Check sheet for the drawn part. Datum: minimum x, y, z corner. Units: mm. A direction names the side the tool comes from. Give positions to 0.01 mm unless a question says otherwise; leave off trailing zeros. Order: outer loops, then holes, each group sorted by start corner. A loop starts at its lowest first (then second) coordinate and runs counter-clockwise, first axis right, second up. Notation, with made-up numbers: M 0,80.5 L 31,80.5 A32 cw 31,117.5 Z; hole C -17.75,-17 d7. An arc over 180 degrees is marked long. Put each result on its own line as item: value. Start each with the question number.
Q1. Section check C-C on z = 8. Record the cut outline in (x, y), then the cut area to 3 significant figures.
Q2. Section check B-B on x = 14. Record the cut outline in (y, z), then the cut area to 3 significant figures.
Q3. Access from +Z, -Z, +X, -X, +Y, -Y to the whole of each face (thin tool, end or side, straight path). Record for the marked faces 5 and 6.
Q4. Mould release check, pull along Z, two halves, no side actions. Record for the marked faces 1, 2, 3 and 4: +Z half, -Z half, draft (parallel to the pull), parting line (faces both ways), or undercut.
Q5. Material ranges on L1, parallel to X at y = 9, z = 23.25; L2, parallel to Y at x = 14, z = 27.05; L3, parallel to X at y = 2.5, z = 14.75, recorded low to high.
Q6. Section check A-A on z = 19.25. Record the cut outline in (x, y).
Q7. Section check D-D on x = 9.75. Record the cut outline in (y, z).
Q8. Go/stop test with a flat-tipped pin: pin 1 (6 mm diameter, centred on x = 12.5, z = 22, fed in from -Y). Record where the tip stops, or that it passes through.
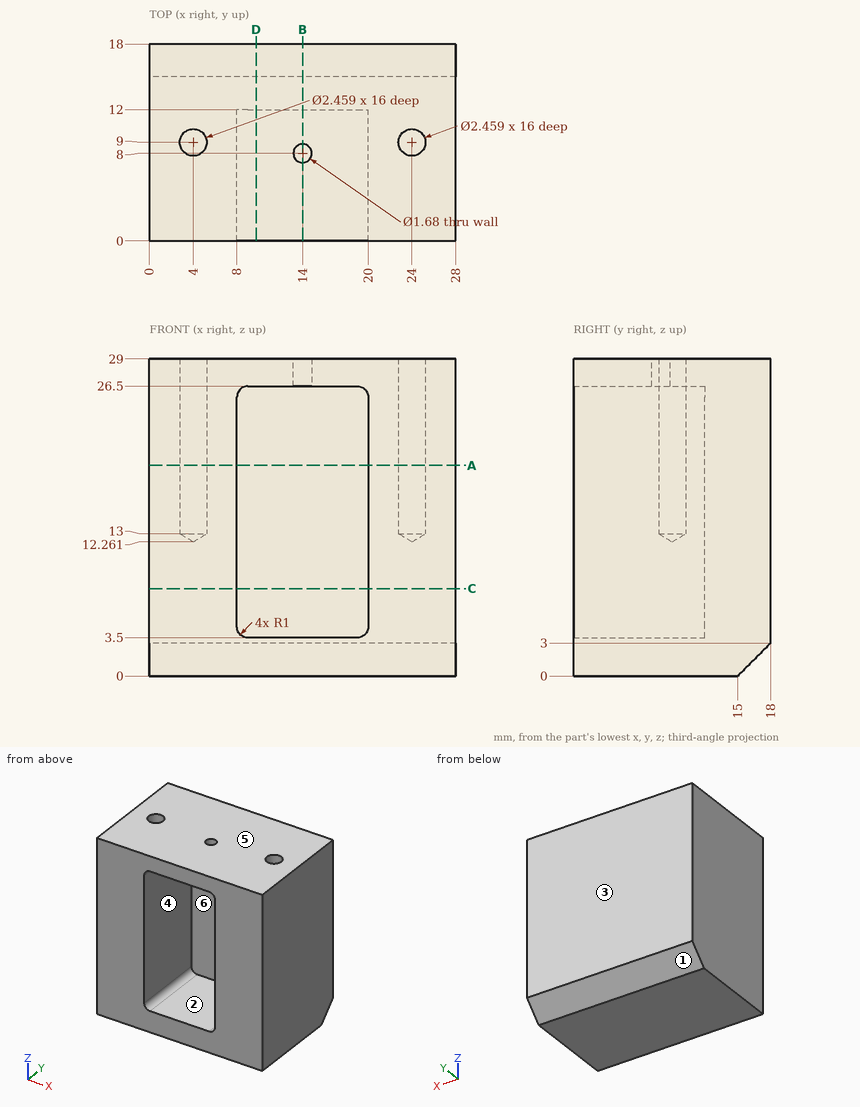
Results found:
1. outline: M 0,0 L 8,0 L 8,12 L 20,12 L 20,0 L 28,0 L 28,18 L 0,18 Z
1. area: 360 mm^2
2. outline: M 0,0 L 15,0 L 18,3 L 18,29 L 8.84,29 L 8.84,26.5 L 12,26.5 L 12,3.5 L 0,3.5 Z; M 0,26.5 L 7.16,26.5 L 7.16,29 L 0,29 Z
2. area: 237 mm^2
3. face 5: +Z, +X, -X, +Y, -Y
3. face 6: -Y
4. face 1: -Z half
4. face 2: undercut
4. face 3: draft
4. face 4: undercut
5. L1: x = 0 to 2.77, 5.23 to 8, 20 to 22.77, 25.23 to 28
5. L2: y = 0 to 7.16, 8.84 to 18
5. L3: x = 0 to 8, 20 to 28
6. outline: M 0,0 L 8,0 L 8,12 L 20,12 L 20,0 L 28,0 L 28,18 L 0,18 Z; hole C 4,9 d2.46; hole C 24,9 d2.46
7. outline: M 0,0 L 15,0 L 18,3 L 18,29 L 0,29 L 0,26.5 L 12,26.5 L 12,3.5 L 0,3.5 Z
8. pin 1: stops at y = 12
